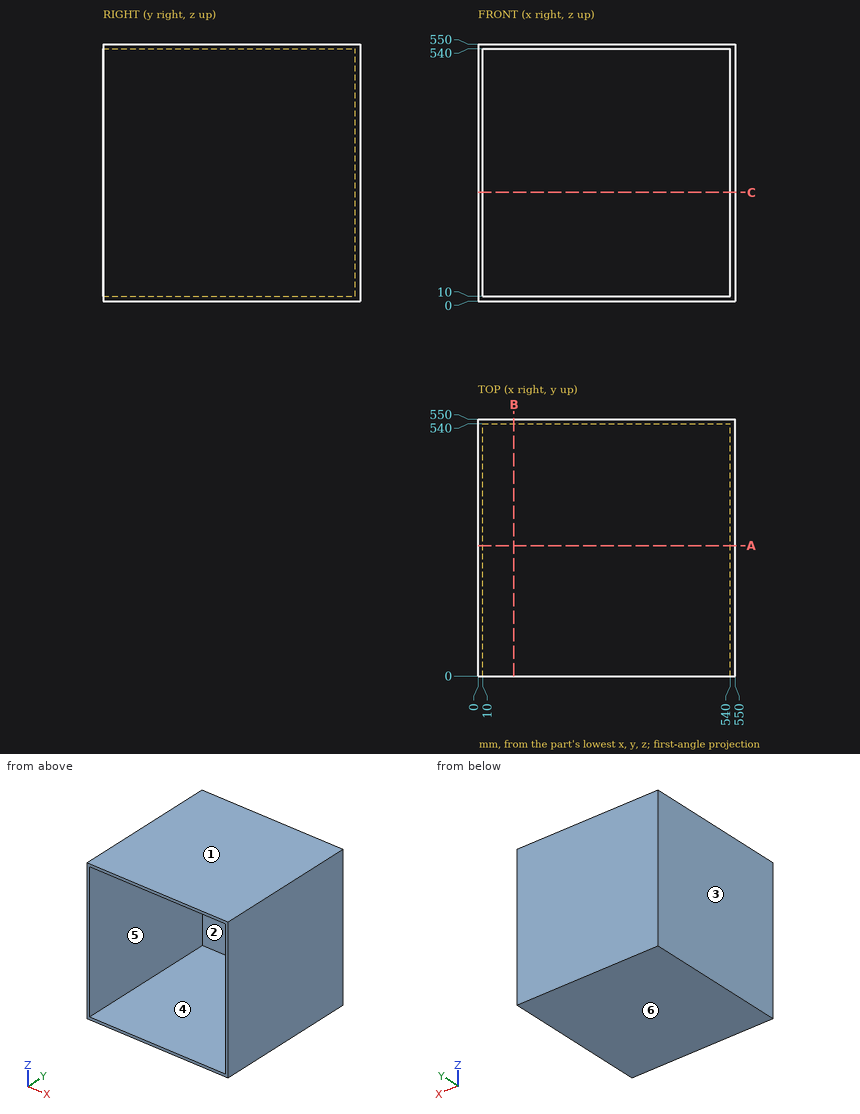
Study the drawing (mm; zero at the part's minimum x, y, z) and answer. A direction names the side the tool comes from. Give positions to 0.01 mm unless a question says otherwise; leave off trailing zeros. Order: outer loops, then holes, each group sorted by start corner. A loop starts at its lowest first (then second) coordinate and runs counter-clockwise, first axis right, second up.
1. Section C-C, the plane z = 232.5 is taken. Determine the outline of the cut face in (x, y), and give its area (3 significant figures).
Result sheet:
outline: (0, 0) - (10, 0) - (10, 540) - (540, 540) - (540, 0) - (550, 0) - (550, 550) - (0, 550) - close
area: 16,300 mm2
2. Straight lines are drawn through the part: L1, parallel to Z at x = 319, y = 48; L2, parallel to Y at x = 384, z = 37.5. For each, find the intervals that lie inside material, in ascending order.
Result sheet:
L1: z = 0 to 10, 540 to 550
L2: y = 540 to 550
3. The mould has two halves that part along X. Classify the marked faces 3, 4, 5 and 6: released by +X, released by -X, zero draft, split by the parting line, or undercut.
Result sheet:
face 3: released by -X
face 4: undercut
face 5: undercut
face 6: zero draft
4. Section A-A, the plane y = 279 is taken. Determine the outline of the cut face in (x, z).
Result sheet:
outline: (0, 0) - (550, 0) - (550, 550) - (0, 550) - close; hole (10, 10) - (540, 10) - (540, 540) - (10, 540) - close
5. Section B-B, the plane x = 76.5 is taken. Determine the outline of the cut face in (y, z), and give its area (3 significant figures).
Result sheet:
outline: (0, 0) - (550, 0) - (550, 550) - (0, 550) - (0, 540) - (540, 540) - (540, 10) - (0, 10) - close
area: 16,300 mm2
6. For the marked faces 1 and 2, determine the directions among +Z, -Z, +X, -X, +Y, -Y from which every point of the face is accessible in a straight line to the end or side of a thin tool.
Result sheet:
face 1: +Z, +X, -X, +Y, -Y
face 2: -Y
